```python
from build123d import *

# Parameters (mm, degrees)
SKETCH1_R           = 7.2
BOSS_EXTRUDE1_DEPTH = 4.5
BOSS_EXTRUDE3_DEPTH = 1


with BuildPart() as part:
    # Sketch1 → Boss-Extrude1 (new body)
    with BuildSketch(Plane.XY):
        Circle(SKETCH1_R)
    extrude(amount=BOSS_EXTRUDE1_DEPTH)

    # Sketch4 → Boss-Extrude3 (add)
    with BuildSketch(Plane(origin=(0, 0, 0), x_dir=(-1, 0, 0), z_dir=(0, 0, -1))):
        with BuildLine():
            Line((10.7, 1.2), (8.111719916, 1.2))
            ThreePointArc((8.111719916, 1.2), (5.798275606, 5.798275606), (1.2, 8.111719916))
            Line((1.2, 8.111719916), (1.2, 10.7))
            Line((1.2, 10.7), (-1.2, 10.7))
            Line((-1.2, 10.7), (-1.2, 8.111719916))
            ThreePointArc((-1.2, 8.111719916), (-5.798275606, 5.798275606), (-8.111719916, 1.2))
            Line((-8.111719916, 1.2), (-10.7, 1.2))
            Line((-10.7, 1.2), (-10.7, -1.2))
            Line((-10.7, -1.2), (-8.111719916, -1.2))
            ThreePointArc((-8.111719916, -1.2), (-5.798275606, -5.798275606), (-1.2, -8.111719916))
            Line((-1.2, -8.111719916), (-1.2, -10.7))
            Line((-1.2, -10.7), (1.2, -10.7))
            Line((1.2, -10.7), (1.2, -8.111719916))
            ThreePointArc((1.2, -8.111719916), (5.798275606, -5.798275606), (8.111719916, -1.2))
            Line((8.111719916, -1.2), (10.7, -1.2))
            Line((10.7, -1.2), (10.7, 1.2))
        make_face()
    extrude(amount=BOSS_EXTRUDE3_DEPTH)


solid = part.part
```
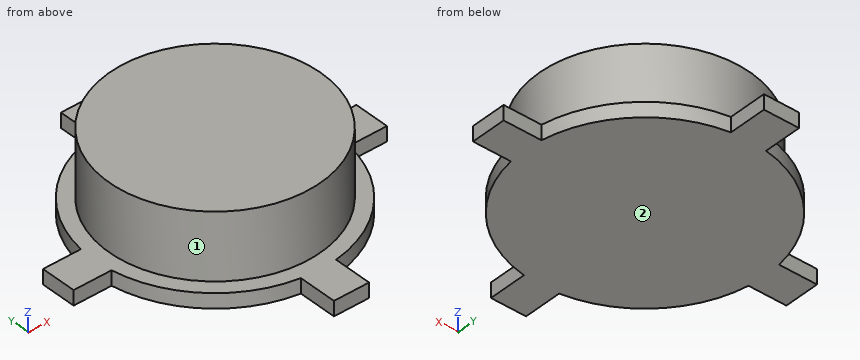
CAD build for the part. Positions are in the model's coordinates, mm. Face numbers are marked on the shaded views. A direction names the side the tool comes from. Round coordinates to 2 decimals unless told otherwise and drop trailing zeros. Write each loop counter-clockwise with the first axis right and the second up, starting at its lowest first coordinate (ties: lowest second). Pieces come first, ordered by that corner, then holes. Notation, with made-up numbers: (-33.75, 49.5) - (-1.75, 49.5) arc R22 cw to (-1.75, 75.5) - close; hole circle Ø4 at (52, -15.75). An arc over 180 degrees is marked (long way). Write item = value, one per line. Start each with the question number.
Q1. Which spindle directions (+Z, -Z, +X, -X, +Y, -Y) get a long thin tool onto all of the face, cutting with end or side? Do the marked faces 1 and 2. Say none if no direction does.
Q2. Band-saw the part on C-C (z = 0.6). Give the cut face in (x, y).
Q3. Band-saw the part on A-A (x = 0). Give the cut face in (y, z).
Q4. Probe L1, parallel to Z at x = -7, y = -2.5; L2, parallel to X at y = -4.25, z = 0.9; L3, parallel to X at y = -3.5, z = 1.25. List the from-to ranges inside material, lowest first. Write a range as from..to.
Q5. Drop flat-ended pins along their axis: pin 1 (0.5 mm diameter, centred on y = 10, z = -0.5, fed in from +X); pin 2 (1.1 mm diameter, centred on x = -9.5, z = -0.5, fed in from +Y); pin 3 (1 mm diameter, centred on y = 3.5, z = 3, fed in from +X). Give the stop position or say it passes through.
Q6. Band-saw the part on D-D (x = 8.75). Give the cut face in (y, z).
Answers below:
q1.face_1 = +Z
q1.face_2 = -Z, +X, -X, +Y, -Y
q2.outline = circle Ø14.4 at (0, 0)
q3.outline = (-10.7, -1) - (10.7, -1) - (10.7, 0) - (7.2, 0) - (7.2, 4.5) - (-7.2, 4.5) - (-7.2, 0) - (-10.7, 0) - close
q4.L1 = -1..0
q4.L2 = -5.81..5.81
q4.L3 = -6.29..6.29
q5.pin_1 = 1.2
q5.pin_2 = 1.2
q5.pin_3 = 6.55
q6.outline = (-1.2, -1) - (1.2, -1) - (1.2, 0) - (-1.2, 0) - close
